Geometry check sheet. Reference: the model listing, model coordinates, mm. A direction names the side the tool comes from. Give positions to 0.01 mm unless a question says otherwise; leave off trailing zeros. Order: outer loops, then holes, each group sorted by start corner. A loop starts at its lowest first (then second) coordinate and runs counter-clockwise, first axis right, second up. Notation, with made-up numbers: M 63,38 L 80,38 A17 cw 80,66 Z; hole C 7.25,-17.5 d9. An arc over 180 degrees is marked long. Answer as CSV lines item,"result".
Autodesk Inventor part; units mm, degrees
ref_plane "YZ Plane" through (0, 0, 0) normal (1, 0, 0) x (0, 1, 0)
ref_plane "XZ Plane" through (0, 0, 0) normal (0, 1, 0) x (-1, 0, 0)
ref_plane "XY Plane" through (0, 0, 0) normal (0, 0, 1) x (1, 0, 0)
sketch "Sketch1" plane through (0, 0, 0) normal (0, 1, 0) x (-1, 0, 0)
  circle A0 centre (0, 0) radius 2.9
  dimension "d0" = 5.8
extrude "Extrusion1" add sketch "Sketch1" along normal blind 1
sketch "Sketch2" plane through (0, 1, 0) normal (0, 1, 0) x (1, 0, 0)
  circle A0 centre (0, 0) radius 1.5
  dimension "d3" = 3
extrude "Extrusion2" add sketch "Sketch2" along normal blind 6
sketch "Sketch3" plane through (0, 0, 0) normal (0, -1, 0) x (1, 0, 0)
  line L0 (0, -1.1547) -> (-1, -0.5774)
  line L1 (-1, -0.5774) -> (-1, 0.5774)
  line L2 (-1, 0.5774) -> (0, 1.1547)
  line L3 (0, 1.1547) -> (1, 0.5774)
  line L4 (1, 0.5774) -> (1, -0.5774)
  line L5 (1, -0.5774) -> (0, -1.1547)
  point P0 (0, 0)
  point P1 (0, 0)
  dimension "d6" = 2
extrude "Extrusion3" cut sketch "Sketch3" against normal blind 1
properties part number "m3_bolt_pan_8mm" material "Stainless Steel"
(1) Draft check along Z on faces 4 (the face through (0, 7, 0)), 5 (the face through (-1.5, 3.96, 0.07)), 6 (the face through (0.51, 0.49, -0.86)). Enter one of: +Z half, -Z half, draft (parallel to the pull), parting line (faces both ways), or undercut.
The answers:
face 4,"draft"
face 5,"parting line"
face 6,"undercut"
(2) Section check B-B on x = -2.1. Enter the section's corners in (y, z).
The answers:
outline,"M 0,-2 L 1,-2 L 1,2 L 0,2 Z"
(3) Section check A-A on z = 0. Enter the section's corners in (x, y).
The answers:
outline,"M -2.9,0 L -1,0 L -1,1 L 1,1 L 1,0 L 2.9,0 L 2.9,1 L 1.5,1 L 1.5,7 L -1.5,7 L -1.5,1 L -2.9,1 Z"
(4) Gauge pin test, flat ends, axial feed: P1, Ø1.5, axis at x = 2, y = 3, coming from the -Z side; P2, Ø2, axis at x = 1.5, z = 0, coming from the -Y side; P3, Ø3, axis at x = -1, y = 5.5, coming from the +Z side; P4, Ø2, axis at x = 2, y = 4.5, coming from the +Z side. Record the tip position at first contact, or that the pin passes through.
The answers:
P1,"stops at z = -0.83"
P2,"stops at y = 0"
P3,"stops at z = 1.5"
P4,"stops at z = 1.12"
(5) Material ranges on line 1 (Y direction, x = -0.7, z = 2.3); line 2 (Y direction, x = -0.25, z = -0.3); line 3 (Z direction, x = -0.05, y = 6), recorded low to high.
The answers:
line 1,"y = 0 to 1"
line 2,"y = 1 to 7"
line 3,"z = -1.5 to 1.5"
(6) Tool access check on faces 1 (the face through (0, 1, 0)), 2 (the face through (-1.2, 1, -1.2)), 3 (the face through (-1.2, 0, 0)). Record the directions out of +Z, -Z, +X, -X, +Y, -Y that give a thin tool (end or side, any length) a straight path to the whole face; none if there is none.
The answers:
face 1,"-Y"
face 2,"+Y"
face 3,"+Z, -Z, +X, -X, -Y"
(7) Section check D-D on x = -0.15. Enter the section's corners in (y, z), then the cut area to 3 significant figures.
The answers:
outline,"M 0,-2.9 L 1,-2.9 L 1,-1.49 L 7,-1.49 L 7,1.49 L 1,1.49 L 1,2.9 L 0,2.9 L 0,1.07 L 1,1.07 L 1,-1.07 L 0,-1.07 Z"
area,"21.6 mm2"
(8) Section check C-C on y = 2. Enter the section's corners in (x, z).
The answers:
outline,"C 0,0 d3"
